Part print with two shaded views. Sizes in mm from the minimum x, y, z corner. Give positions to 0.01 mm unless a question says otherwise; leave off trailing zeros. Write each loop counter-clockwise with the first axis right and the second up, starting at its lowest first coordinate (ties: lowest second). Pieces come first, ordered by that corner, then holes. Notation, with made-up numbers: (50.25, -23) - (80.25, -23) arc R27 cw to (80.25, 14) - close; hole circle Ø3 at (-22.5, 11). An arc over 180 degrees is marked (long way). Answer as a JSON object with one key per item and string values.
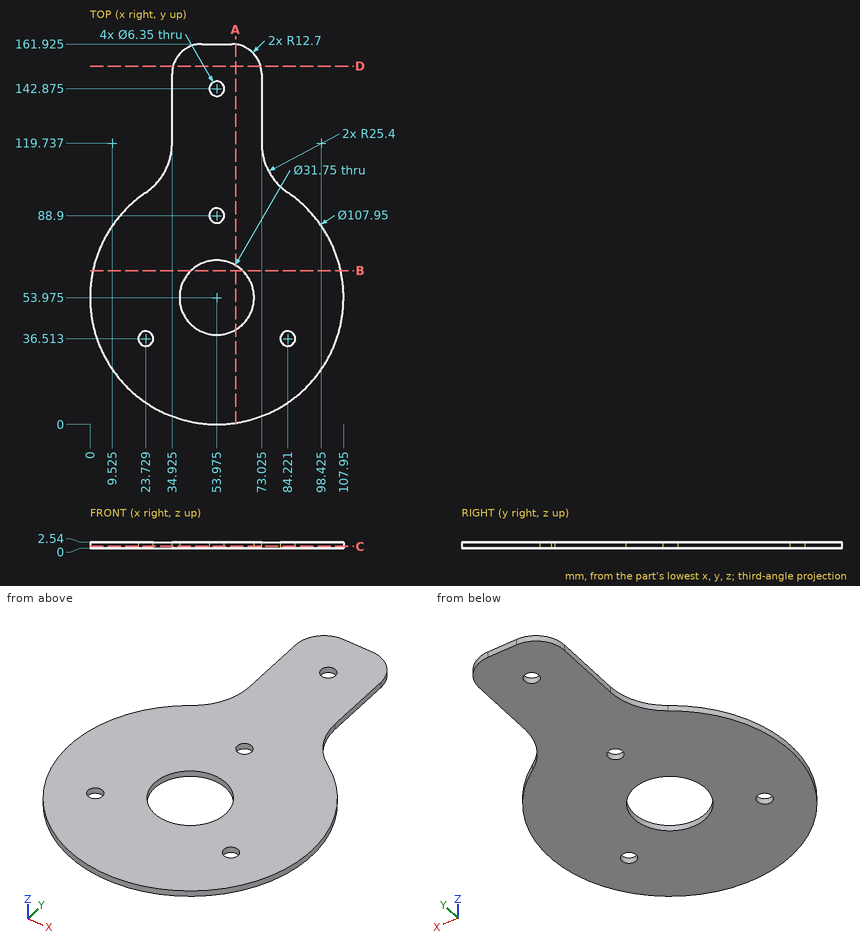
(1) Saw through at B-B, the plane y = 65.5. Give the cut face in (x, z) (1 decimal).
Answer key:
{"outline": "(1.2, 0) - (43.1, 0) - (43.1, 2.5) - (1.2, 2.5) - close; (64.9, 0) - (106.7, 0) - (106.7, 2.5) - (64.9, 2.5) - close"}
(2) Probe L1, parallel to X at y = 35, z = 0.7 (1 decimal); L2, parallel to X at y = 57, z = 1 (1 decimal); L3, parallel to X at y = 143.5, z = 2 (1 decimal). List the from-to ranges inside material, lowest first. Write a range as [from, to].
Answer key:
{"L1": "x = [3.4, 20.9], [26.5, 81.4], [87, 104.5]", "L2": "x = [0.1, 38.4], [69.6, 107.9]", "L3": "x = [34.9, 50.9], [57.1, 73]"}
(3) Saw through at D-D, the plane y = 152.5. Give the cut face in (x, z) (1 decimal).
Answer key:
{"outline": "(35.4, 0) - (72.6, 0) - (72.6, 2.5) - (35.4, 2.5) - close"}
(4) Flat gauge pins, fed straight in: P1, Ø4, axis at x = 84.22, y = 36.51, coming from the +Z side; P2, Ø1.3, axis at y = 136.5, z = 1, coming from the +X side (1 decimal); P3, Ø1, axis at y = 33, z = 0.5, coming from the -X side (1 decimal); P4, Ø1, axis at x = 94.5, z = 1, coming from the -Y side (1 decimal). Where does each tip first touch, or does it go through?
Answer key:
{"P1": "passes through", "P2": "stops at x = 73", "P3": "stops at x = 4", "P4": "stops at y = 17.8"}
(5) Saw through at C-C, the plane z = 0.85. State how many separate pieces and enclosed holes the cut face has, and give its area (3 significant figures).
Answer key:
{"separate pieces": "1", "enclosed holes": "5", "area": "10,300 mm²"}
(6) Saw through at A-A, the plane x = 62. Give the cut face in (y, z) (1 decimal), and give its area (3 significant figures).
Answer key:
{"outline": "(0.6, 0) - (40.3, 0) - (40.3, 2.5) - (0.6, 2.5) - close; (67.7, 0) - (161.8, 0) - (161.8, 2.5) - (67.7, 2.5) - close", "area": "340 mm²"}
